from build123d import *

# Parameters (mm, degrees)
SKETCH1_R           = 14.0975
BOSS_EXTRUDE1_DEPTH = 11
SKETCH4_R           = 14.0975
BOSS_EXTRUDE2_DEPTH = 2.25
SKETCH5_R           = 10.4
CUT_EXTRUDE1_DEPTH  = 2.25
SKETCH3_W           = 10.575
SKETCH3_H           = 12.228258218
CUT_EXTRUDE5_DEPTH  = 8.75
SKETCH6_R           = 3
CUT_EXTRUDE6_DEPTH  = 9
FILLET5_R           = 2.25
FILLET6_R           = 2.25


with BuildPart() as part:
    # Sketch1 → Boss-Extrude1 (new body)
    with BuildSketch(Plane(origin=(0, 0, 0), x_dir=(1, 0, 0), z_dir=(0, 1, 0))):
        with BuildLine():
            Line((-17.7875, -22.628070726), (17.7875, -22.628070726))
            Line((17.7875, -22.628070726), (17.7875, 0))
            ThreePointArc((17.7875, 0), (0, 17.7875), (-17.7875, 0))
            Line((-17.7875, 0), (-17.7875, -22.628070726))
        make_face()
        with Locations(Location((0, 0, 0), (0, 0, 270))):
            Circle(SKETCH1_R, mode=Mode.SUBTRACT)
    extrude(amount=BOSS_EXTRUDE1_DEPTH)

    # Sketch4 → Boss-Extrude2 (add)
    with BuildSketch(Plane.XZ):
        with Locations(Location((0, 0, 0), (0, 0, 270))):
            Circle(SKETCH4_R)
    extrude(amount=-BOSS_EXTRUDE2_DEPTH)

    # Sketch5 → Cut-Extrude1 (cut)
    with BuildSketch(Plane(origin=(0, 2.25, 0), x_dir=(1, 0, 0), z_dir=(0, 1, 0))):
        with Locations(Location((0, 0, 0), (0, 0, 270))):
            Circle(SKETCH5_R)
    extrude(amount=-CUT_EXTRUDE1_DEPTH, mode=Mode.SUBTRACT)

    # Sketch3 → Cut-Extrude5 (cut)
    with BuildSketch(Plane(origin=(0, 11, 0), x_dir=(1, 0, 0), z_dir=(0, 1, 0))):
        with Locations((0, -16.513941617)):
            Rectangle(SKETCH3_W, SKETCH3_H)
    extrude(amount=-CUT_EXTRUDE5_DEPTH, mode=Mode.SUBTRACT)

    # Sketch6 → Cut-Extrude6 (cut)
    with BuildSketch(Plane.XY.offset(22.628070726)):
        with Locations((-12.2875, 5.5)):
            Circle(SKETCH6_R)
        with Locations((12.2875, 5.5)):
            Circle(SKETCH6_R)
    extrude(amount=-CUT_EXTRUDE6_DEPTH, mode=Mode.SUBTRACT)

    # Fillet5
    fillet5_edges = [part.edges().sort_by_distance(p)[0] for p in [
        (17.7875, 0, 11.314035363),
        (-17.7875, 0, 11.314035363),
        (0, 0, -17.7875),
    ]]
    fillet(fillet5_edges, radius=FILLET5_R)

    # Fillet6
    fillet6_edges = [part.edges().sort_by_distance(p)[0] for p in [
        (17.7875, 11, 11.314035363),
        (0, 11, -17.7875),
        (-17.7875, 11, 11.314035363),
    ]]
    fillet(fillet6_edges, radius=FILLET6_R)


solid = part.part
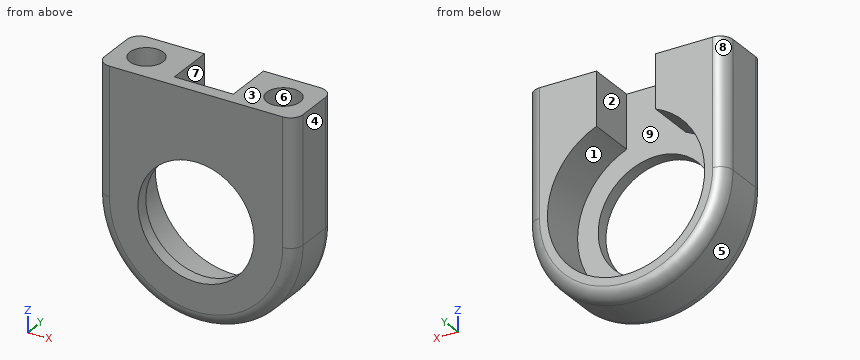
Geometry: final body of the model. Coordinates: model frame, mm. Face numbers are marked on the shaded views. A direction names the side the tool comes from. Give positions to 0.01 mm unless a question says otherwise; leave off trailing zeros. Write each loop counter-clockwise with the first axis right and the second up, starting at its lowest first coordinate (ties: lowest second). Pieces come first, ordered by that corner, then holes.
(1) Mould query, pull axis X, two halves, no side actions, for the marked faces 1, 2, 3 and 4. Classes: released by +X, released by -X, zero draft, split by the parting line, or undercut.
(2) Cut plane D-D, the plane z = 9. Return loops of the section in (x, y).
(3) First-contact query: P1, Ø5, axis at x = -12.29, y = 5.5, coming from the -Z side; P2, Ø12, axis at x = 8, z = 4, coming from the -Y side; P3, Ø5, axis at y = 6, z = -6, coming from the -X side; P4, Ø4, axis at y = 6, z = -7, coming from the -X side. Flat tips, straight axial feed; report the tip coordinate or a pass-through.
(4) Cut plane B-B, the plane z = 16. Return loops of the section in (x, y).
(5) Cut plane C-C, the plane y = 5.5. Return loops of the section in (x, z) (1 decimal).
(6) Ray query, line 1 (X direction, y = 5.75, z = 14.5); line 2 (X direction, y = 4, z = 15.5); line 3 (Y direction, x = -3, z = 13). Return the intervals inside material, ascending.
(7) Cut plane A-A, the plane x = 0. Return loops of the section in (y, z), then the cut area to 3 significant figures.
(8) Access query for the marked faces 5, 6, 7, 8 and 9. Directions: +Z, -Z, +X, -X, +Y, -Y. A direction counts if a zero-diameter tool reaches every point of the face in a straight line with its end or side. Return the directions, or none.
Values follow:
1. face 1: undercut
1. face 2: undercut
1. face 3: zero draft
1. face 4: released by +X
2. outline: (-17.79, 2.25) arc R2.25 ccw to (-15.54, 0) - (-5.21, 0) - (-5.21, 2.25) - (-10.85, 2.25) - (-10.85, 11) - (-15.54, 11) arc R2.25 ccw to (-17.79, 8.75) - close; (5.21, 0) - (15.54, 0) arc R2.25 ccw to (17.79, 2.25) - (17.79, 8.75) arc R2.25 ccw to (15.54, 11) - (10.85, 11) - (10.85, 2.25) - (5.21, 2.25) - close
3. P1: stops at z = -14.85
3. P2: stops at y = 0
3. P3: stops at x = -17.44
3. P4: stops at x = -17.07
4. outline: (-17.79, 2.25) arc R2.25 ccw to (-15.54, 0) - (15.54, 0) arc R2.25 ccw to (17.79, 2.25) - (17.79, 8.75) arc R2.25 ccw to (15.54, 11) - (5.29, 11) - (5.29, 2.25) - (-5.29, 2.25) - (-5.29, 11) - (-15.54, 11) arc R2.25 ccw to (-17.79, 8.75) - close; hole circle Ø6 at (-12.29, 5.5); hole circle Ø6 at (12.29, 5.5)
5. outline: (-17.8, 0) arc R17.8 ccw to (17.8, 0) - (17.8, 22.6) - (15.3, 22.6) - (15.3, 13.6) - (9.3, 13.6) - (9.3, 22.6) - (5.3, 22.6) - (5.3, 13.1) arc R14.1 cw (long way) to (-5.3, 13.1) - (-5.3, 22.6) - (-9.3, 22.6) - (-9.3, 13.6) - (-15.3, 13.6) - (-15.3, 22.6) - (-17.8, 22.6) - close
6. line 1: x = -17.79 to -15.28, -9.3 to -5.29, 5.29 to 9.3, 15.28 to 17.79
6. line 2: x = -17.79 to -14.89, -9.69 to -5.29, 5.29 to 9.69, 14.89 to 17.79
6. line 3: y = 0 to 2.25
7. outline: (0, -15.54) arc R2.25 ccw to (2.25, -17.79) - (8.75, -17.79) arc R2.25 ccw to (11, -15.54) - (11, -14.1) - (2.25, -14.1) - (2.25, -10.4) - (0, -10.4) - close; (0, 10.4) - (2.25, 10.4) - (2.25, 22.63) - (0, 22.63) - close
7. area: 74.2 mm2
8. face 5: -Z, +Y, -Y
8. face 6: +Z
8. face 7: +Z, +Y
8. face 8: +Z, -Z, -X, +Y
8. face 9: +Y
